```python
from build123d import *

# Parameters (mm, degrees)
F0_W          = 110.617
F0_H          = 110.617
F1_DEPTH      = 53.721
F1_DEPTH_BACK = 53.721
F2_R          = 38.1
F3_DEPTH      = 54.229
F4_R          = 38.1
F5_DEPTH      = 54.229


with BuildPart() as f1:
    # F0 (on Top) → F1 (new body, two sides)
    with BuildSketch(Plane.XY) as f1_sk:
        with Locations((55.3085, -55.3085)):
            Rectangle(F0_W, F0_H)
    extrude(amount=F1_DEPTH)
    extrude(f1_sk.sketch, amount=-F1_DEPTH_BACK)

    # F2 (on face) → F3 (join)
    with BuildSketch(Plane.XY.offset(53.721)):
        with Locations((55.3085, -55.3085)):
            Circle(F2_R)
    extrude(amount=F3_DEPTH)

    # F4 (on face) → F5 (join)
    with BuildSketch(Plane(origin=(0, 0, -53.721), x_dir=(1, 0, 0), z_dir=(0, 0, -1))):
        with Locations((55.3085, 55.3085)):
            Circle(F4_R)
    extrude(amount=F5_DEPTH)


solid = f1.part
```
For this review, take the finished solid that the model builds, in its own axes (mm). A direction names the side the tool comes from. Round coordinates to 2 decimals unless told otherwise and drop trailing zeros. Write each loop counter-clockwise with the first axis right and the second up, starting at its lowest first coordinate (ties: lowest second). Pieces come first, ordered by that corner, then holes. Notation, with made-up numbers: (85, 32.5) - (134, 32.5) arc R7 ccw to (134, 36.5) - close; hole circle Ø10 at (42.5, 38.5). An arc over 180 degrees is marked (long way). Put each result on its own line as item: value.
Q1. Insertion check: pin 1 Ø3 at (x, y) = (58.5, -97.5) entering from -Z; pin 2 Ø1 at (y, z) = (-50, -82.5) entering from +X; pin 3 Ø2 at (x, z) = (75.5, -58.5) entering from -Y. Each pin has a flat end and moves straight along its axis. Give the tip position at first contact, or say it passes through.
Solved:
pin 1: stops at z = -53.72
pin 2: stops at x = 93.1
pin 3: stops at y = -88.22
Q2. Wall thickness on probe 1 along Z at (x, y) = (95, -35); probe 2 along Y at (x, z) = (52.5, 60.5); probe 3 along Y at (x, z) = (80, -93): over which ranges is each line inside the solid? List them lowest first.
Solved:
probe 1: z = -53.72 to 53.72
probe 2: y = -93.3 to -17.31
probe 3: y = -84.32 to -26.29
Q3. We need section B-B (x = 79.5). Give the boundary of the cut face in (y, z).
Solved:
outline: (-110.62, -53.72) - (-84.74, -53.72) - (-84.74, -107.95) - (-25.87, -107.95) - (-25.87, -53.72) - (0, -53.72) - (0, 53.72) - (-25.87, 53.72) - (-25.87, 107.95) - (-84.74, 107.95) - (-84.74, 53.72) - (-110.62, 53.72) - close
Q4. We need section D-D (y = -12.5). Give the boundary of the cut face in (x, z).
Solved:
outline: (0, -53.72) - (110.62, -53.72) - (110.62, 53.72) - (0, 53.72) - close
Q5. Mouldability with a two-part tool opening along Y and no side actions: class faces 4 (the face through (72.889, -21.507, -80.456)), 5 (the face through (110.617, -56, 1)), 6 (the face through (55, -110.617, 1)) as released by +Y, released by -Y, zero draft, split by the parting line, or undercut.
Solved:
face 4: split by the parting line
face 5: zero draft
face 6: released by -Y
Q6. We need section C-C (z = 83). Give the boundary of the cut face in (x, y).
Solved:
outline: circle Ø76.2 at (55.31, -55.31)
Q7. Machinability: for faces 1 (the face through (18, -42, -53.721)), 2 (the face through (55, 0, 1)), 3 (the face through (91.649, -43.864, 80.456)), which of the approach directions +Z, -Z, +X, -X, +Y, -Y give a long, thin tool a straight path to every point of the face, cutting with its end or side? Answer none if there is none.
Solved:
face 1: -Z
face 2: +Z, -Z, +X, -X, +Y
face 3: +Z
Q8. We need section A-A (y = -82). Give the boundary of the cut face in (x, z), and give its area (3 significant figures).
Solved:
outline: (0, -53.72) - (28.12, -53.72) - (28.12, -107.95) - (82.5, -107.95) - (82.5, -53.72) - (110.62, -53.72) - (110.62, 53.72) - (82.5, 53.72) - (82.5, 107.95) - (28.12, 107.95) - (28.12, 53.72) - (0, 53.72) - close
area: 17,800 mm2
